```python
from build123d import *

# Parameters (mm, degrees)
CROQUIS1_R              = 23.6
SALIENTE_EXTRUIR1_DEPTH = 8
VACIADO1_T              = 5
CORTAR_EXTRUIR1_START   = -214
CROQUIS2_R              = 23.6
CORTAR_EXTRUIR1_DEPTH   = 214


with BuildPart() as part:
    # Croquis1 → Saliente-Extruir1 (new body)
    with BuildSketch(Plane(origin=(0, 0, 0), x_dir=(0, 0, -1), z_dir=(1, 0, 0))):
        with BuildLine():
            Line((165, -35), (165, 35))
            ThreePointArc((165, 35), (150.355339059, 70.355339059), (115, 85))
            add(Edge.make_bspline(
                [(-115, 85), (0, 45), (115, 85)],
                knots=[0, 0, 0, 1, 1, 1], degree=2))
            ThreePointArc((-115, 85), (-150.355339059, 70.355339059), (-165, 35))
            Line((-165, 35), (-165, -35))
            ThreePointArc((-165, -35), (-150.355339059, -70.355339059), (-115, -85))
            add(Edge.make_bspline(
                [(-115, -85), (0, -45), (115, -85)],
                knots=[0, 0, 0, 1, 1, 1], degree=2))
            ThreePointArc((115, -85), (150.355339059, -70.355339059), (165, -35))
        make_face()
        with Locations((-100, 0)):
            Circle(CROQUIS1_R, mode=Mode.SUBTRACT)
    extrude(amount=SALIENTE_EXTRUIR1_DEPTH)

    # Vaciado1
    vaciado1_openings = [part.faces().sort_by_distance(p)[0] for p in [
        (8, 0, -3.797931414),
    ]]
    offset(amount=VACIADO1_T, openings=vaciado1_openings, kind=Kind.INTERSECTION)

    # Croquis2 → Cortar-Extruir1 (cut)
    with BuildSketch(Plane(origin=(8, 0, 0), x_dir=(0, 0, -1), z_dir=(1, 0, 0)).offset(CORTAR_EXTRUIR1_START)):
        with Locations((-100, 0)):
            Circle(CROQUIS2_R)
    extrude(amount=CORTAR_EXTRUIR1_DEPTH, mode=Mode.SUBTRACT)


solid = part.part
```
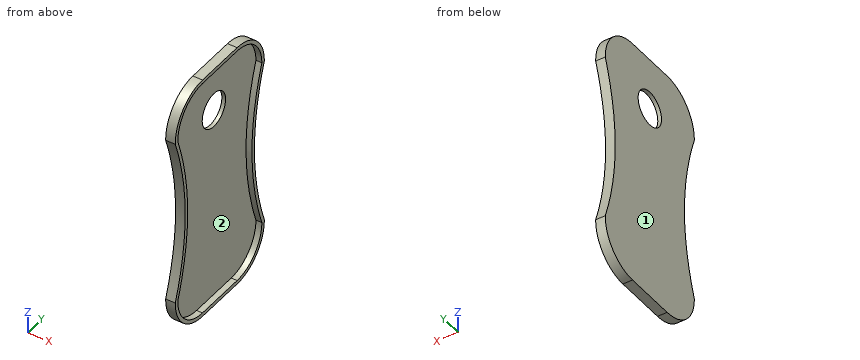
Check sheet for the modelled part. Datum: model origin and axes. Units: mm. Face numbers are marked on the shaded views. Give positions to 0.01 mm unless a question says otherwise; leave off trailing zeros. Order: outer loops, then holes, each group sorted by start corner. A loop starts at its lowest first (then second) coordinate and runs counter-clockwise, first axis right, second up. Notation, with made-up numbers: M 19,13.25 L 39,13.25 A30 ccw 39,35.25 Z; hole C -23,21.25 d4. An arc over 180 degrees is marked long. Answer in a Markdown table with one row per item. Add a question column.
Q1. Sectioned sample at A-A, the plane y = 0. Record the boundary of the cut face in (x, z).
Q2. Sectioned sample at C-C, the plane y = 45. Record the boundary of the cut face in (x, z), and give its area (3 significant figures).
Q3. Gauge pin test, flat ends, axial feed: pin 1 Ø1 at (x, z) = (-1.5, -109) entering from -Y; pin 2 Ø1.5 at (x, y) = (4, -38.5) entering from +Z; pin 3 Ø4 at (x, y) = (-0.5, -38.5) entering from +Z. Record the tip position at first contact, or that the pin passes through.
Q4. Sectioned sample at B-B, the plane z = -128.5. Record the boundary of the cut face in (x, y).
Q5. Thickness scan on L1, parallel to Z at x = 4.75, y = -35; L2, parallel to Z at x = -3.9, y = 0; L3, parallel to Y at x = 6, z = 127.5. Record the ranges inside material, lowest first.
Q6. Release check for a two-part mould opening along Z. For the marked faces 1 and 2 record: released by +Z, released by -Z, zero draft, split by the parting line, or undercut.
Verdict:
| question | item | result |
|---|---|---|
| 1 | outline | M -5,-170 L 8,-170 L 8,-165 L 0,-165 L 0,76.4 L -5,76.4 Z; M -5,123.6 L 0,123.6 L 0,165 L 8,165 L 8,170 L -5,170 Z |
| 2 | outline | M -5,-169.08 L 8,-169.08 L 8,-163.99 L 0,-163.99 L 0,163.99 L 8,163.99 L 8,169.08 L -5,169.08 Z |
| 2 | area | 1,770 mm² |
| 3 | pin 1 | y = -88.4 |
| 3 | pin 2 | z = 169.93 |
| 3 | pin 3 | z = 169.98 |
| 4 | outline | M -5,-88.32 L 8,-88.32 L 8,-83.14 L 0,-83.14 L 0,83.14 L 8,83.14 L 8,88.32 L -5,88.32 Z |
| 5 | L1 | -170 to -165, 165 to 170 |
| 5 | L2 | -170 to 76.4, 123.6 to 170 |
| 5 | L3 | -88.56 to -83.41, 83.41 to 88.56 |
| 6 | face 1 | zero draft |
| 6 | face 2 | undercut |
